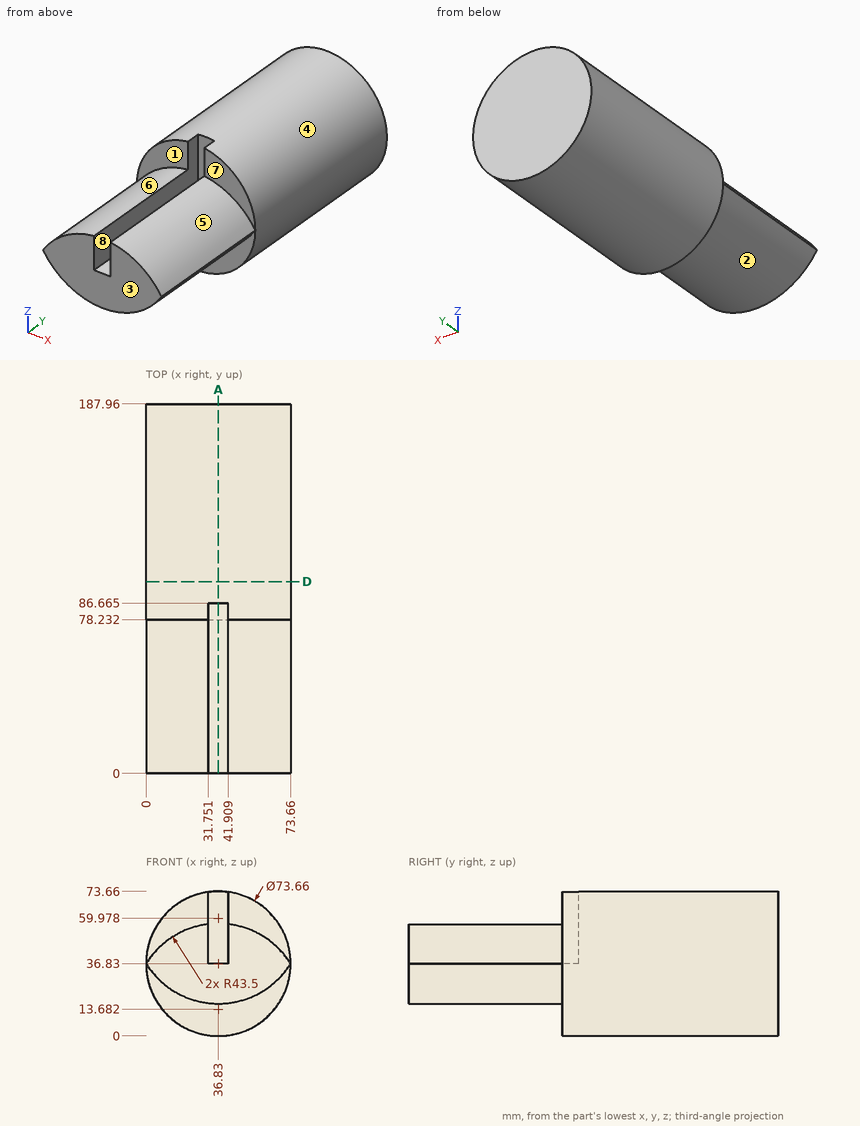
Check sheet for the drawn part. Datum: minimum x, y, z corner. Units: mm. A direction names the side the tool comes from. Round coordinates to 2 decimals unless told otherwise and drop trailing zeros. Order: outer loops, then holes, each group sorted by start corner. A loop starts at its lowest first (then second) coordinate and runs counter-clockwise, first axis right, second up.
1) Section check D-D (y = 97.5). Record the boundary of the cut face in (x, z), and give its area (3 significant figures).
2) Mould release check, pull along X, two halves, no side actions. Record for the marked faces 6, 7 and 8: +X half, -X half, draft (parallel to the pull), parting line (faces both ways), or undercut.
3) Section check A-A (x = 36.83). Record the boundary of the cut face in (y, z) (1 decimal).
4) Tool access check on the marked faces 1, 2, 3, 4 and 5. Record the directions out of +Z, -Z, +X, -X, +Y, -Y that give a thin tool (end or side, any length) a straight path to the whole face; none if there is none.
5) Scan lines: line 1 (Y direction, x = 67.5, z = 28.5); line 2 (X direction, y = 81, z = 62.5); line 3 (Z direction, x = 31, y = 177) (1 decimal). Record each from-to range of solid material in increasing order.
6) Go/stop test with flat-tipped pins: pin 1 Ø1 at (x, y) = (49.5, 133.5) entering from +Z; pin 2 Ø4 at (x, y) = (64, 92) entering from +Z; pin 3 Ø10 at (x, y) = (60, 30.5) entering from +Z (1 decimal). Record where each tip stops, or that it passes through.
Result:
1. outline: circle Ø73.66 at (36.83, 36.83)
1. area: 4,260 mm2
2. face 6: -X half
2. face 7: draft
2. face 8: undercut
3. outline: (0, 16.5) - (78.2, 16.5) - (78.2, 0) - (188, 0) - (188, 73.7) - (86.7, 73.7) - (86.7, 36.8) - (0, 36.8) - close
4. face 1: +Z, -X, -Y
4. face 2: -Z, -Y
4. face 3: +Z, -Z, +X, -X, -Y
4. face 4: +Y, -Y
4. face 5: +Z, +X, -Y
5. line 1: y = 78.23 to 187.96
5. line 2: x = 10.42 to 31.75, 41.91 to 63.24
5. line 3: z = 0.5 to 73.2
6. pin 1: stops at z = 71.59
6. pin 2: stops at z = 63.72
6. pin 3: stops at z = 53.2
